```python
from build123d import *

# Parameters (mm, degrees)
SKETCH1_W               = 38.1
SKETCH1_H               = 38.1
SKETCH1_W_2             = 33.3756
SKETCH1_H_2             = 33.3756
EXTRUDE1_DEPTH          = 431.8
F_1_4_CLEARANCE_HOLE1_D = 7.14248
F_3_8_CLEARANCE_HOLE1_D = 10.0838


with BuildPart() as part:
    # Sketch1 → Extrude1 (new body)
    with BuildSketch(Plane.XY):
        Rectangle(SKETCH1_W, SKETCH1_H)
        Rectangle(SKETCH1_W_2, SKETCH1_H_2, mode=Mode.SUBTRACT)
    extrude(amount=EXTRUDE1_DEPTH)

    # 1/4 Clearance Hole1 (through all)
    with Locations(Plane(origin=(19.05, 0, 358.775), x_dir=(0, 1, 0), z_dir=(1, 0, 0))):
        with Locations((0, 0), (0, -44.45), (0, -288.925), (0, -333.375)):
            Hole(F_1_4_CLEARANCE_HOLE1_D / 2)

    # 3/8 Clearance Hole1 (through all)
    with Locations(Plane(origin=(19.05, 0, 419.1), x_dir=(0, 1, 0), z_dir=(1, 0, 0))):
        with Locations((0, 0), (0, -158.75)):
            Hole(F_3_8_CLEARANCE_HOLE1_D / 2)


solid = part.part
```
CAD build for the part. Positions are in the model's coordinates, mm. A direction names the side the tool comes from. Round coordinates to 2 decimals unless told otherwise and drop trailing zeros. Loops run counter-clockwise (first coordinate to the right, second up) from the corner with the lowest first, then second, coordinate; pieces in that order, holes last. Notation, with made-up numbers: M -13,-31 L 31,-31 A19 cw 31,5 Z; hole C 23.5,77.5 d11. An arc over 180 degrees is marked long. Use a Markdown table: item, result. Add a question column.
(1) Flat gauge pin, fed straight in: pin 1 (12 mm diameter, centred on x = -8, y = 5, fed in from +Z). Where does the tip first touch, or does it go through?
(2) Cut at D-D (z = 126). Give the cut face in (x, y), and give its area (3 significant figures).
(3) Drill centre lines: line 1 (X direction, y = 15, z = 319); line 2 (Y direction, x = -18, z = 69). Where is each one in solid material? Low to high.
(4) Cut at B-B (z = 69.85). Give the cut face in (x, y).
(5) Cut at A-A (y = -10). Give the cut face in (x, z), and give its area (3 significant figures).
(6) Which spindle directions (+Z, -Z, +X, -X, +Y, -Y) get a long thin tool onto all of the face, cutting with end or side? Do faces 4 (the face through (0, -16.688, 213)), 5 (the face through (19.05, 0, 213)). Say none if no direction does.
(7) Pull direction Z, two halves, no side cores. Call faces 1 (the face through (16.688, 0, 213)), 2 (the face through (-17, 0, 0)), 3 (the face through (-17.89, 0.46, 28.94)): +Z half, -Z half, draft (parallel to the pull), parting line (faces both ways), or undercut.
Geometry says:
| question | item | result |
|---|---|---|
| 1 | pin 1 | passes through |
| 2 | outline | M -19.05,-19.05 L 19.05,-19.05 L 19.05,19.05 L -19.05,19.05 Z; hole M -16.69,-16.69 L 16.69,-16.69 L 16.69,16.69 L -16.69,16.69 Z |
| 2 | area | 338 mm² |
| 3 | line 1 | x = -19.05 to -16.69, 16.69 to 19.05 |
| 3 | line 2 | y = -19.05 to -3.47, 3.47 to 19.05 |
| 4 | outline | M -19.05,-19.05 L 19.05,-19.05 L 19.05,-3.57 L 16.69,-3.57 L 16.69,-16.69 L -16.69,-16.69 L -16.69,-3.57 L -19.05,-3.57 Z; M -19.05,3.57 L -16.69,3.57 L -16.69,16.69 L 16.69,16.69 L 16.69,3.57 L 19.05,3.57 L 19.05,19.05 L -19.05,19.05 Z |
| 5 | outline | M -19.05,0 L -16.69,0 L -16.69,431.8 L -19.05,431.8 Z; M 16.69,0 L 19.05,0 L 19.05,431.8 L 16.69,431.8 Z |
| 5 | area | 2,040 mm² |
| 6 | face 4 | +Z, -Z |
| 6 | face 5 | +Z, -Z, +X, +Y, -Y |
| 7 | face 1 | draft |
| 7 | face 2 | -Z half |
| 7 | face 3 | undercut |
